Design review of the part built by this model. Coordinates are the model's own, in mm. A direction names the side the tool comes from. Round coordinates to 2 decimals unless told otherwise and drop trailing zeros. Loops run counter-clockwise (first coordinate to the right, second up) from the corner with the lowest first, then second, coordinate; pieces in that order, holes last. Notation, with made-up numbers: (42.5, 88) -> (88.5, 88) arc R17 ccw to (88.5, 109) -> close; hole circle Ø6 at (-22, 22). An arc over 180 degrees is marked (long way). Answer as CSV lines item,"result". Start each with the question number.
(1) Take a section at B-B, the plane z = 0.4. Write out the cut boundary in (x, y), and give its area (3 significant figures).
(2) Take a section at A-A, the plane x = 25. Write out the cut boundary in (y, z), and give its area (4 significant figures).
(3) Take a section at C-C, the plane y = -31. Write out the cut boundary in (x, z), and give its area (3 significant figures).
(4) Draft analysis for pull direction Y (two halves, no side actions). For faces 4 (the face through (28, -39, 1)), 5 (the face through (14.8, -38.9, 0.7)), 6 (the face through (34, -35, 1)), state which applies: +Y half, -Y half, draft (parallel to the pull), parting line (faces both ways), or undercut.
(5) For P1, Ø0.8, axis at x = 3.5, z = 1, coming from the -Y side, flat-tipped, find the tip position at first contact; note if it passes through.
(6) To check wall thickness, follow line 1 (X direction, y = -11, z = 1.4); line 2 (Y direction, x = 22, z = 0.65); line 3 (X direction, y = -8, z = 1.3). State the ranges of each line that lie inside material, in increasing order. Write a range as from..to.
(7) Machinability: for faces 1 (the face through (14.5, -10, 1)), 2 (the face through (10, -39, 1)), 3 (the face through (29, -36, 1)), which of the approach directions +Z, -Z, +X, -X, +Y, -Y give a long, thin tool a straight path to every point of the face, cutting with its end or side? Answer none if there is none.
(8) Take a section at D-D, the plane y = -38. Write out the cut boundary in (x, z).
from build123d import *

# Parameters (mm, degrees)
SZKIC1_R                    = 1.5
SZKIC1_R_2                  = 1.822392888
DODANIE_WYCI_GNI_CIE1_DEPTH = 1.5
SFAZOWANIE1_SIZE            = 2


with BuildPart() as part:
    # Szkic1 → Dodanie-wyciągnięcie1 (new body)
    with BuildSketch(Plane.XY):
        Polygon((0, 0), (38, 0), (38, -35), (31.060112688, -35), (28, -35), (28, -40.397059959), (28, -41), (10, -41), (10, -40.699902364), (10, -35), (5.889298893, -35), (0, -35), align=None)
        with Locations((16, -38)):
            Circle(SZKIC1_R, mode=Mode.SUBTRACT)
        with Locations((22, -38)):
            Circle(SZKIC1_R, mode=Mode.SUBTRACT)
        with Locations((33, -31)):
            Circle(SZKIC1_R_2, mode=Mode.SUBTRACT)
        with BuildLine():
            Line((26.5, -8.5), (26.5, -11))
            ThreePointArc((26.5, -11), (25, -12.5), (23.5, -11))
            Line((23.5, -11), (23.5, -8.5))
            ThreePointArc((23.5, -8.5), (25, -7), (26.5, -8.5))
        make_face(mode=Mode.SUBTRACT)
        with BuildLine():
            Line((11.5, -8.5), (11.5, -11))
            ThreePointArc((11.5, -11), (13, -12.5), (14.5, -11))
            Line((14.5, -11), (14.5, -8.5))
            ThreePointArc((14.5, -8.5), (13, -7), (11.5, -8.5))
        make_face(mode=Mode.SUBTRACT)
    extrude(amount=DODANIE_WYCI_GNI_CIE1_DEPTH)

    # Sfazowanie1
    sfazowanie1_edges = [part.edges().sort_by_distance(p)[0] for p in [
        (28, -35, 0.75),
        (10, -35, 0.75),
    ]]
    chamfer(sfazowanie1_edges, length=SFAZOWANIE1_SIZE)


solid = part.part
The answers:
1,outline,"(0, -35) -> (8, -35) -> (10, -37) -> (10, -41) -> (28, -41) -> (28, -37) -> (30, -35) -> (38, -35) -> (38, 0) -> (0, 0) -> close; hole (11.5, -11) arc R1.5 ccw to (14.5, -11) -> (14.5, -8.5) arc R1.5 ccw to (11.5, -8.5) -> close; hole circle Ø3 at (16, -38); hole circle Ø3 at (22, -38); hole (23.5, -11) arc R1.5 ccw to (26.5, -11) -> (26.5, -8.5) arc R1.5 ccw to (23.5, -8.5) -> close; hole circle Ø3.64 at (33, -31)"
1,area,"1,390 mm²"
2,outline,"(-41, 0) -> (-12.5, 0) -> (-12.5, 1.5) -> (-41, 1.5) -> close; (-7, 0) -> (0, 0) -> (0, 1.5) -> (-7, 1.5) -> close"
2,area,"53.25 mm²"
3,outline,"(0, 0) -> (31.18, 0) -> (31.18, 1.5) -> (0, 1.5) -> close; (34.82, 0) -> (38, 0) -> (38, 1.5) -> (34.82, 1.5) -> close"
3,area,"51.5 mm²"
4,face 4,"draft"
4,face 5,"undercut"
4,face 6,"-Y half"
5,P1,"y = -35"
6,line 1,"0..11.5, 14.5..23.5, 26.5..38"
6,line 2,"-41..-39.5, -36.5..0"
6,line 3,"0..11.59, 14.41..23.59, 26.41..38"
7,face 1,"+Z, -Z"
7,face 2,"+Z, -Z, -X, -Y"
7,face 3,"+Z, -Z, +X, -Y"
8,outline,"(10, 0) -> (14.5, 0) -> (14.5, 1.5) -> (10, 1.5) -> close; (17.5, 0) -> (20.5, 0) -> (20.5, 1.5) -> (17.5, 1.5) -> close; (23.5, 0) -> (28, 0) -> (28, 1.5) -> (23.5, 1.5) -> close"
